The model under review builds one solid part; all positions refer to its coordinate system, in mm. Face numbers are marked on the shaded views. A direction names the side the tool comes from. Coordinates: 2 decimals unless noted, no trailing zeros. Write each loop counter-clockwise with the first axis right and the second up, starting at its lowest first coordinate (ties: lowest second). Pieces come first, ordered by that corner, then holes. Notation, with made-up numbers: (23.25, -1) - (75.25, -1) arc R20 cw to (75.25, 23) - close; hole circle Ø11 at (77.5, 0.5). An arc over 180 degrees is marked (long way). Return JSON: item names as keys, results as strings. Group by question number.
(1) Tool access review of the marked faces 1 and 2: name each direction out of +Z, -Z, +X, -X, +Y, -Y from which nothing blocks a thin tool from reaching the whole face with its end or side.
(2) For pin 1 Ø1.5 at (x, z) = (-123, 149) entering from +Y; pin 2 Ø4 at (y, z) = (2.5, -177) entering from +X; pin 3 Ø5 at (y, z) = (2, -116) entering from +X, all flat-tipped, find the tip position at first contact; note any pin that passes through.
(3) We need section B-B on z = 0. State the section outline as (x, y) points.
(4) We need section A-A on x = 0. State the section outline as (y, z) points.
(5) To check wall thickness, follow L1, parallel to X at y = 1.4, z = 0; L2, parallel to Y at x = -180, z = 99.5; L3, parallel to Z at x = 195, y = -2. State the ranges of each line that lie inside material, in increasing order. Write a range as from..to.
(6) Draft analysis for pull direction X (two halves, no side actions). For the marked faces 3 and 4, state which applies: released by +X, released by -X, zero draft, split by the parting line, or undercut.
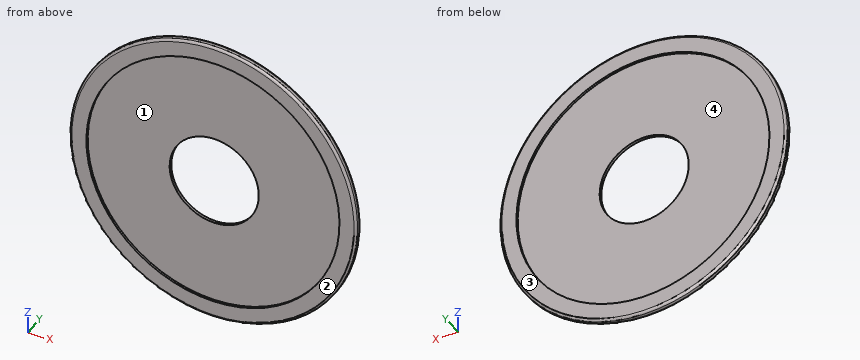
```python
from build123d import *

# Parameters (mm, degrees)
SKETCH1_W = 165.1
SKETCH1_H = 4.7625


with BuildPart() as part:
    # Sketch1 → Revolve1 (revolve)
    with BuildSketch(Plane.XY, mode=Mode.PRIVATE) as revolve1_sk:
        with Locations((158.75, 2.38125)):
            Rectangle(SKETCH1_W, SKETCH1_H)
    revolve(revolve1_sk.sketch.rotate(Axis((0, -187.080769231, 0), (0, 1, 0)), 90), axis=Axis((0, -187.080769231, 0), (0, 1, 0)))

    # Sketch2 → Revolve2 (revolve)
    with BuildSketch(Plane.XY, mode=Mode.PRIVATE) as revolve2_sk:
        with BuildLine():
            Line((216.3, -3.81), (241.3, -3.81))
            ThreePointArc((241.3, -3.81), (243.994076836, -2.694076836), (245.11, 0))
            Line((245.11, 0), (245.11, 4.7625))
            ThreePointArc((245.11, 4.7625), (243.994076836, 7.456576836), (241.3, 8.5725))
            Line((241.3, 8.5725), (216.3, 8.5725))
            Line((216.3, 8.5725), (216.3, 4.7625))
            Line((216.3, 4.7625), (241.3, 4.7625))
            Line((241.3, 4.7625), (241.3, 0))
            Line((241.3, 0), (216.3, 0))
            Line((216.3, 0), (216.3, -3.81))
        make_face()
    revolve(revolve2_sk.sketch.rotate(Axis((0, 0, 0), (0, 1, 0)), 90), axis=Axis((0, 0, 0), (0, 1, 0)))


solid = part.part
```
Ans:
{
 "1": {"face 1": "-Y", "face 2": "+Z, -Z, +X, -X, -Y"},
 "2": {"pin 1": "y = 4.76", "pin 2": "x = 171.62", "pin 3": "x = 217.25"},
 "3": {"outline": "(-245.11, 0) arc R3.81 ccw to (-241.3, -3.81) - (-216.3, -3.81) - (-216.3, 0) - (-76.2, 0) - (-76.2, 4.76) - (-216.3, 4.76) - (-216.3, 8.57) - (-241.3, 8.57) arc R3.81 ccw to (-245.11, 4.76) - close; (76.2, 0) - (216.3, 0) - (216.3, -3.81) - (241.3, -3.81) arc R3.81 ccw to (245.11, 0) - (245.11, 4.76) arc R3.81 ccw to (241.3, 8.57) - (216.3, 8.57) - (216.3, 4.76) - (76.2, 4.76) - close"},
 "4": {"outline": "(-3.81, -241.3) arc R3.81 ccw to (0, -245.11) - (4.76, -245.11) arc R3.81 ccw to (8.57, -241.3) - (8.57, -216.3) - (4.76, -216.3) - (4.76, -76.2) - (0, -76.2) - (0, -216.3) - (-3.81, -216.3) - close; (-3.81, 216.3) - (0, 216.3) - (0, 76.2) - (4.76, 76.2) - (4.76, 216.3) - (8.57, 216.3) - (8.57, 241.3) arc R3.81 ccw to (4.76, 245.11) - (0, 245.11) arc R3.81 ccw to (-3.81, 241.3) - close"},
 "5": {"L1": "-245.11..-76.2, 76.2..245.11", "L2": "0..4.76", "L3": "-147.57..-93.6, 93.6..147.57"},
 "6": {"face 3": "zero draft", "face 4": "undercut"}
}
